```python
from build123d import *

# Parameters (mm, degrees)
EXTRUDE_1_DEPTH     = 6
SKETCH_2_W          = 250
SKETCH_2_H          = 250
CUT_EXTRUDE_1_DEPTH = 1361.160284672
SKETCH_3_W          = 80
SKETCH_3_H          = 250
CUT_EXTRUDE_2_DEPTH = 10


with BuildPart() as part:
    # 草图1 → 凸台-拉伸1 (new body)
    with BuildSketch(Plane.XY):
        Polygon((0, -100), (0, 800), (1100, 800), (1100, 600), (90, -100), align=None)
    extrude(amount=EXTRUDE_1_DEPTH)

    # 草图2 → 切除-拉伸1 (cut, through all)
    with BuildSketch(Plane.XY.offset(6)):
        with Locations((365, 675)):
            Rectangle(SKETCH_2_W, SKETCH_2_H)
    extrude(amount=-CUT_EXTRUDE_1_DEPTH, mode=Mode.SUBTRACT)

    # 草图3 → 切除-拉伸2 (cut)
    with BuildSketch(Plane.XY.offset(6)):
        with Locations((530, 675)):
            Rectangle(SKETCH_3_W, SKETCH_3_H)
    extrude(amount=-CUT_EXTRUDE_2_DEPTH, mode=Mode.SUBTRACT)


solid = part.part
```
Geometry check sheet. Reference: the model listing, model coordinates, mm. Give positions to 0.01 mm unless a question says otherwise; leave off trailing zeros. Loops run counter-clockwise (first coordinate to the right, second up) from the corner with the lowest first, then second, coordinate; pieces in that order, holes last. Notation, with made-up numbers: M 55,3.5 L 109,3.5 A24 ccw 109,34.5 Z; hole C 65,2 d11. An arc over 180 degrees is marked long. Write item = value, one per line.
(1) Sectioned sample at A-A, the plane z = 4.3. Record the cut outline in (x, y), plus the area to 3 significant figures.
Answer below:
outline = M 0,-100 L 90,-100 L 1100,600 L 1100,800 L 570,800 L 570,550 L 240,550 L 240,800 L 0,800 Z
area = 554,000 mm2
(2) Gauge pin test, flat ends, axial feed: pin 1 Ø3 at (y, z) = (8.5, 3.5) entering from +X; pin 2 Ø1 at (x, z) = (752, 5.5) entering from -Y. Record the tip position at first contact, or that the pin passes through.
Answer below:
pin_1 = 248.71
pin_2 = 358.47
(3) Material ranges on line 1 (X direction, y = 714.5, z = 2.9); line 2 (Y direction, x = 838.5, z = 5.4); line 3 (Y direction, x = 960, z = 2.25), recorded low to high. Write a range as [from, to].
Answer below:
line_1 = [0, 240], [570, 1100]
line_2 = [418.76, 800]
line_3 = [502.97, 800]
(4) Sectioned sample at C-C, the plane x = 405. Record the cut outline in (y, z), plus the area to 3 significant figures.
Answer below:
outline = M 118.32,0 L 550,0 L 550,6 L 118.32,6 Z
area = 2,590 mm2
(5) Sectioned sample at B-B, the plane y = 100.5. Record the cut outline in (x, z), plus the area to 3 significant figures.
Answer below:
outline = M 0,0 L 379.29,0 L 379.29,6 L 0,6 Z
area = 2,280 mm2
